Could you check a few things on this model? Use its own coordinates, in mm. A direction names the side the tool comes from. Coordinates: 2 decimals unless noted, no trailing zeros. Order: outer loops, then holes, each group sorted by start corner. A loop starts at its lowest first (then second) coordinate and runs counter-clockwise, first axis right, second up. Notation, with made-up numbers: (46.5, 15) - (100.5, 15) arc R14 ccw to (100.5, 31) - close; hole circle Ø8 at (69.25, -26.5). An arc over 180 degrees is marked (long way). Answer as a JSON object with one key per item and string values. Group by question number.
(1) Imagine slicing it at B-B, the plane x = 57.5. Write out the boundary of the cut face in (y, z).
(2) Will these pins go through, and if not, where does the flat tip stop? P1, Ø5, axis at y = -10.5, z = 14, coming from the +X side; P2, Ø3, axis at y = -10.5, z = 17.5, coming from the +X side; P3, Ø4, axis at x = 24, z = 33, coming from the -Y side; P4, Ø1, axis at x = 18.5, y = -39, coming from the +Z side.
(3) Imagine slicing it at C-C, the plane z = 10. Write out the boundary of the cut face in (x, y).
(4) Imagine slicing it at A-A, the plane y = -45. Write out the boundary of the cut face in (x, z).
(5) Which directions (+Z, -Z, +X, -X, +Y, -Y) give clear straight access to the entire face, cutting with the end or side of a thin tool? Please do faces 1 (the flat face through (-50, -50, 5)), 2 (the cylindrical face through (1.451, -65.984, 23.734)), 3 (the flat face through (50, -50, 5)), 4 (the cylindrical face through (6.241, -46.354, 2.535)).
(6) We'd pull the mould along Z, two halves only. Please class faces 5 (the flat face through (-16, -47, 43)), 6 (the flat face through (-10, -48, 40)), 7 (the cylindrical face through (-36.07, -20.45, 2.54)): pulls with the +Z half, pulls with the -Z half, needs draft (parallel to the pull), parting line crosses it, or undercut.
(7) Imagine slicing it at D-D, the plane y = -28.5. Write out the boundary of the cut face in (x, z), and give its area (3 significant figures).
(8) Please list where these lines run through material, in increasing order: probe 1 along Z at (x, y) = (13.5, -53); probe 2 along Y at (x, z) = (10, 1.1); probe 3 along Z at (x, y) = (-0.5, -30).
Autodesk Fusion 360 part; units mm, degrees
sketch "Sketch1" plane through (0, 0, 0) normal (0, 0, 1) x (1, 0, 0)
  line L0 (66, 0) -> (-66, 0)
  arc A0 (-66, 0) -> (66, 0) centre (0, 0) ccw
  arc A1 (-63, 0) -> (63, 0) centre (0, 0) ccw
  line L1 (0, -66) -> (-66, -66)
  line L2 (-66, 0) -> (-66, -66)
  circle A2 centre (-57.5, -57.5) radius 2
  line L3 (0, 1.75) -> (0, 22.5)
  line L4 (66, 0) -> (66, -66)
  circle A3 centre (57.5, -57.5) radius 2
  line L5 (0, -66) -> (66, -66)
  arc A4 (-48, 0) -> (48, 0) centre (0, 0) ccw
  circle A5 centre (-10, -8.5) radius 2
  circle A6 centre (10, -8.5) radius 2
  arc A7 (-35.7911, -20) -> (35.7911, -20) centre (0, 0) ccw
  line L6 (-43.6348, -20) -> (-35.7911, -20)
  line L7 (35.7911, -20) -> (43.6348, -20)
  line L8 (-5, -40.694) -> (-5, -47.7389)
  line L9 (5, -40.694) -> (5, -47.7389)
  dimension "d2" = 126
  dimension "d4" = 4
  dimension "d7" = -15
  dimension "d9" = 4
  dimension "d10" = 4
  dimension "d11" = 8.5
  dimension "d12" = 8.5
  dimension "d13" = 56
  dimension "d14" = 56
extrude "Extrude1" add sketch "Sketch1" along normal blind 5 contours L0 A0 A1 | A0 L4 L5 | L0 A1 A4 | A0 L1 L2 | L0 A4 A7 L6 L7 | A4 A7 L8 L9
fillet "Fillet2" radius 3.5 8 edges at (35.7911, -20, 2.5) (43.6348, -20, 2.5) (5, -47.7389, 2.5) (5, -40.694, 2.5) (-43.6348, -20, 2.5) (-35.7911, -20, 2.5) (-5, -40.694, 2.5) (-5, -47.7389, 2.5)
extrude "Extrude2" add sketch "Sketch1" along normal blind 40 contours L0 A0 A1
extrude "Extrude3" add sketch "Sketch1" along normal blind 43 and the other way blind -40 contours L0 A0 A1 | L0 A1 A4
fillet "Fillet1" radius 12.5 2 edges at (-66, -66, 2.5) (66, -66, 2.5)
chamfer "Chamfer1" distance 1 angle 45 4 edges at (-11.8647, -7.7768, 5) (8.1353, -7.7768, 5) (-59.3647, -56.7768, 5) (55.6353, -56.7768, 5)
Result set:
{
 "1": {"outline": "(-65.34, 0) - (-59.5, 0) - (-59.5, 4) - (-60.5, 5) - (-65.34, 5) - close; (-55.5, 0) - (0, 0) - (0, 5) - (-25.74, 5) - (-25.74, 40) - (0, 40) - (0, 43) - (-32.4, 43) - (-32.4, 5) - (-54.5, 5) - (-55.5, 4) - close"},
 "2": {"P1": "stops at x = 65.51", "P2": "stops at x = 65.38", "P3": "stops at y = -62.23", "P4": "passes through"},
 "3": {"outline": "(-66, 0) arc R66 ccw to (66, 0) - (63, 0) arc R63 cw to (-63, 0) - close"},
 "4": {"outline": "(-66, 0) - (-16.7, 0) - (-16.7, 5) - (-44.09, 5) - (-44.09, 40) - (-16.7, 40) - (-16.7, 43) - (-48.28, 43) - (-48.28, 5) - (-66, 5) - close; (-5.26, 0) - (5.26, 0) - (5.26, 5) - (-5.26, 5) - close; (16.7, 0) - (66, 0) - (66, 5) - (48.28, 5) - (48.28, 43) - (16.7, 43) - (16.7, 40) - (44.09, 40) - (44.09, 5) - (16.7, 5) - close"},
 "5": {"face 1": "+Z, -X, -Y", "face 2": "+Z, -Y", "face 3": "+Z, +X, -Y", "face 4": "+Z, -Z"},
 "6": {"face 5": "pulls with the +Z half", "face 6": "undercut", "face 7": "needs draft"},
 "7": {"outline": "(-66, 0) - (-38.62, 0) - (-38.62, 5) - (-56.18, 5) - (-56.18, 40) - (-38.62, 40) - (-38.62, 43) - (-59.53, 43) - (-59.53, 5) - (-66, 5) - close; (-29.47, 0) - (29.47, 0) - (29.47, 5) - (-29.47, 5) - close; (38.62, 0) - (66, 0) - (66, 5) - (59.53, 5) - (59.53, 43) - (38.62, 43) - (38.62, 40) - (56.18, 40) - (56.18, 5) - (38.62, 5) - close", "area": "928 mm^2"},
 "8": {"probe 1": "z = 0 to 5, 40 to 43", "probe 2": "y = -66 to -46.95, -39.76 to -10.5, -6.5 to 0", "probe 3": "z = 0 to 5"}
}
